Answer from the drawing. Dimensions are ordinates in mm from the lowest x, y and z of the part. Give positions to 0.01 mm unless a question says otherwise; leave off trailing zeros. Loops run counter-clockwise (first coordinate to the right, second up) from the corner with the lowest first, then second, coordinate; pieces in that order, holes last.
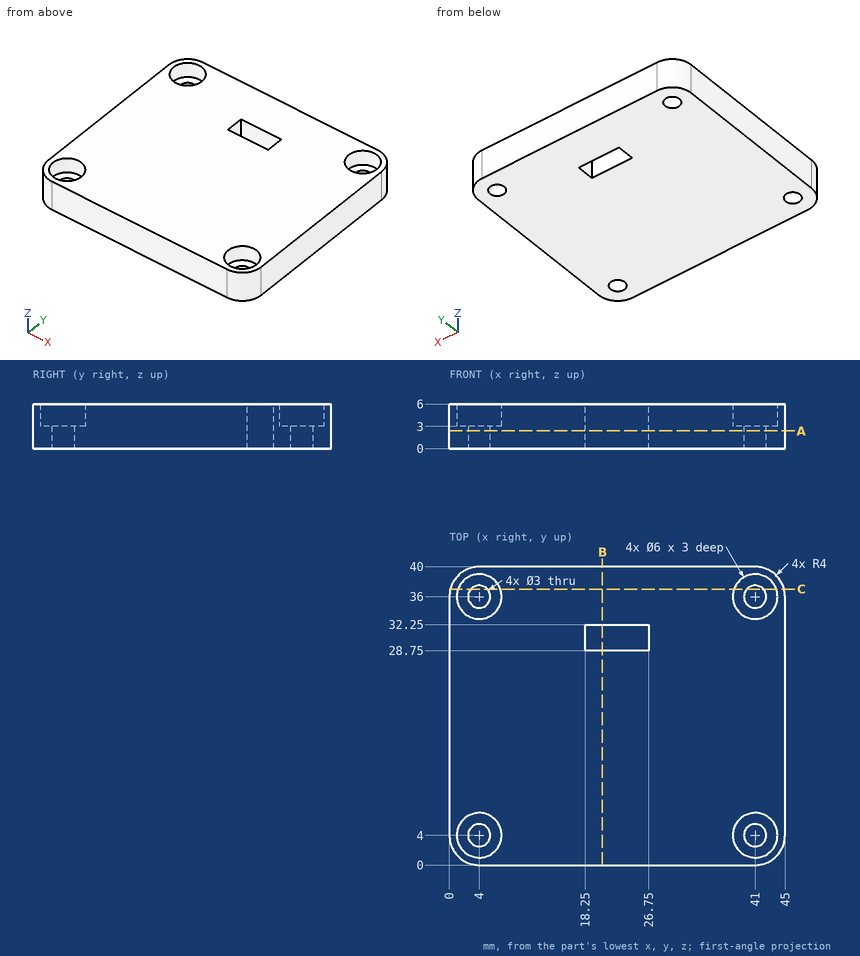
Item 1: Find section C-C, the plane y = 37. Write down the section's boundary in (x, z).
Item 2: Find section B-B, the plane x = 20.5. Write down the section's boundary in (y, z), plus the area to 3 significant figures.
Item 3: Consider line 1 (Y direction, x = 4, z = 3.85); line 2 (X direction, y = 30, z = 2); line 3 (Y direction, x = 19, z = 0.35). Determine where each line is inside the solid, lowest interval first.
Item 4: A flat-ended cylindrical pin translates along its axis: pin 1 Ø3.5 at (x, y) = (4, 4) entering from +Z. Find the tip coordinate at first contact, or state that the pin passes through.
Item 5: Find section A-A, the plane z = 2.4. Write down the section's boundary in (x, y).
Ans:
1. outline: (0.13, 0) - (2.88, 0) - (2.88, 3) - (1.17, 3) - (1.17, 6) - (0.13, 6) - close; (5.12, 0) - (39.88, 0) - (39.88, 3) - (38.17, 3) - (38.17, 6) - (6.83, 6) - (6.83, 3) - (5.12, 3) - close; (42.12, 0) - (44.87, 0) - (44.87, 6) - (43.83, 6) - (43.83, 3) - (42.12, 3) - close
2. outline: (0, 0) - (28.75, 0) - (28.75, 6) - (0, 6) - close; (32.25, 0) - (40, 0) - (40, 6) - (32.25, 6) - close
2. area: 219 mm2
3. line 1: y = 0 to 1, 7 to 33, 39 to 40
3. line 2: x = 0 to 18.25, 26.75 to 45
3. line 3: y = 0 to 28.75, 32.25 to 40
4. pin 1: stops at z = 3
5. outline: (0, 4) arc R4 ccw to (4, 0) - (41, 0) arc R4 ccw to (45, 4) - (45, 36) arc R4 ccw to (41, 40) - (4, 40) arc R4 ccw to (0, 36) - close; hole circle Ø3 at (4, 4); hole circle Ø3 at (4, 36); hole (18.25, 28.75) - (26.75, 28.75) - (26.75, 32.25) - (18.25, 32.25) - close; hole circle Ø3 at (41, 4); hole circle Ø3 at (41, 36)
